For this review, use the dimensioned drawing (mm, ordinates from the lowest corner) and the shaded views. A direction names the side the tool comes from. Round coordinates to 2 decimals unless told otherwise and drop trailing zeros. Loops run counter-clockwise (first coordinate to the right, second up) from the corner with the lowest first, then second, coordinate; pieces in that order, holes last. Notation, with made-up numbers: M 41.25,52.25 L 72.25,52.25 A21 ccw 72.25,72.25 Z; hole C 67,-21 d11. An arc over 180 degrees is marked long. Use a Markdown table: item, result. Add a question column.
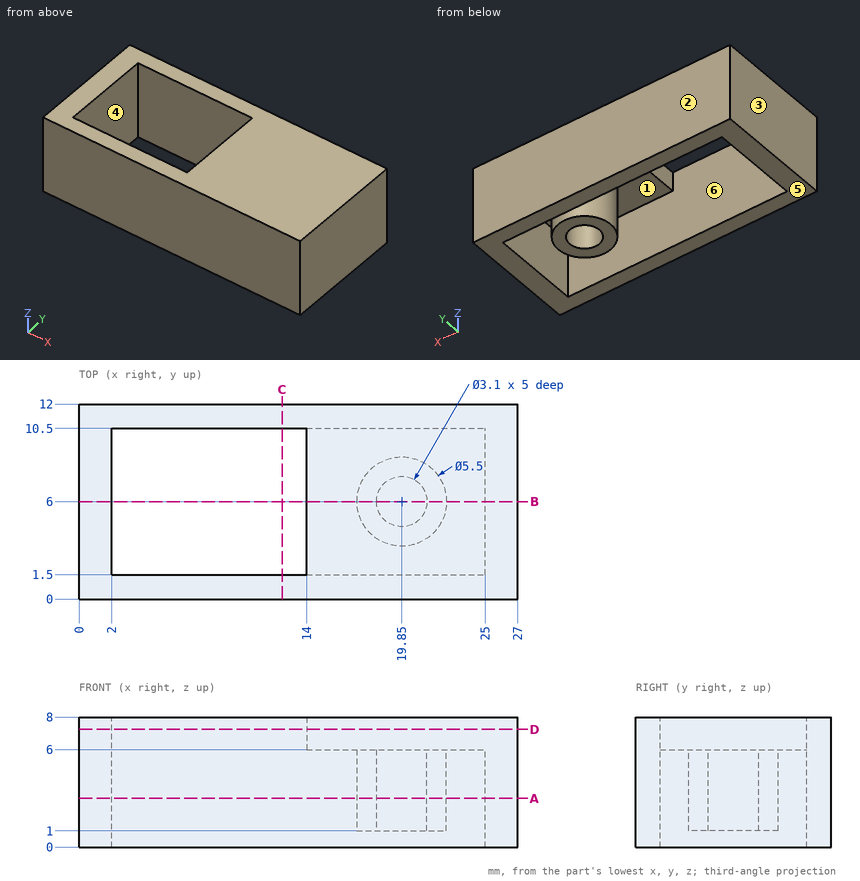
(1) Consider section A-A, the plane z = 3. Give the boundary of the cut face in (x, y), then the cut area to 3 significant figures.
(2) For the marked faces 4, 5 and 6, list the 3-axis set-ups (+Z, -Z, +X, -X, +Y, -Y) from which the entire face can be reached by the end or side of a thin tool; tool diameter is ignored.
(3) Consider section B-B, the plane y = 6. Give the boundary of the cut face in (x, z), then the cut area to 3 significant figures.
(4) Insertion check: pin 1 Ø6 at (x, y) = (15.5, 6.5) entering from -Z; pin 2 Ø1.6 at (x, y) = (20, 6.5) entering from -Z. Each pin has a flat end and moves straight along its axis. Give the tip position at first contact, or say it passes through.
(5) Consider section D-D, the plane z = 7.25. Give the boundary of the cut face in (x, y), then the cut area to 3 significant figures.
(6) Consider section C-C, the plane x = 12.5. Give the boundary of the cut face in (y, z).
(7) Draft analysis for pull direction Y (two halves, no side actions). For the marked faces 1, 2 and 3, state which applies: released by +Y, released by -Y, zero draft, split by the parting line, or undercut.
(8) To check wall thickness, follow probe 1 along Y at (x, z) = (19.85, 3.85); probe 2 along X at (y, z) = (7, 6.5); probe 3 along Y at (x, z) = (10.5, 5.25). State the ranges of each line that lie inside material, in increasing order.
Found:
| question | item | result |
|---|---|---|
| 1 | outline | M 0,0 L 27,0 L 27,12 L 0,12 Z; C 19.85,6 d5.5; hole M 2,1.5 L 25,1.5 L 25,10.5 L 2,10.5 Z; hole C 19.85,6 d3.1 |
| 1 | area | 133 mm^2 |
| 2 | face 4 | +Z, -Z |
| 2 | face 5 | -Z, +X, -X, +Y, -Y |
| 2 | face 6 | -Z |
| 3 | outline | M 0,0 L 2,0 L 2,8 L 0,8 Z; M 14,6 L 17.1,6 L 17.1,1 L 18.3,1 L 18.3,6 L 21.4,6 L 21.4,1 L 22.6,1 L 22.6,6 L 25,6 L 25,0 L 27,0 L 27,8 L 14,8 Z |
| 3 | area | 66.0 mm^2 |
| 4 | pin 1 | stops at z = 1 |
| 4 | pin 2 | stops at z = 6 |
| 5 | outline | M 0,0 L 27,0 L 27,12 L 0,12 Z; hole M 2,1.5 L 14,1.5 L 14,10.5 L 2,10.5 Z |
| 5 | area | 216 mm^2 |
| 6 | outline | M 0,0 L 1.5,0 L 1.5,8 L 0,8 Z; M 10.5,0 L 12,0 L 12,8 L 10.5,8 Z |
| 7 | face 1 | undercut |
| 7 | face 2 | released by +Y |
| 7 | face 3 | zero draft |
| 8 | probe 1 | y = 0 to 1.5, 3.25 to 4.45, 7.55 to 8.75, 10.5 to 12 |
| 8 | probe 2 | x = 0 to 2, 14 to 27 |
| 8 | probe 3 | y = 0 to 1.5, 10.5 to 12 |
